```python
from build123d import *

# Parameters (mm, degrees)
SKETCH1_W         = 18
SKETCH1_H         = 42.5
IDCHAMFER_SIZE    = 2
ODCHAMFER_SIZE    = 4.5
IDCHAMFERFAR_SIZE = 2


with BuildPart() as part:
    # Sketch1 → Base-Revolve (revolve)
    with BuildSketch(Plane.XY, mode=Mode.PRIVATE) as base_revolve_sk:
        with Locations((-9, 103.75)):
            Rectangle(SKETCH1_W, SKETCH1_H)
    revolve(base_revolve_sk.sketch.rotate(Axis((-34.925, 0, 0), (1, 0, 0)), 90), axis=Axis((-34.925, 0, 0), (1, 0, 0)))

    # IDChamfer
    idchamfer_edges = [part.edges().sort_by_distance(p)[0] for p in [
        (0, 0, -82.5),
    ]]
    chamfer(idchamfer_edges, length=IDCHAMFER_SIZE)

    # ODChamfer
    odchamfer_edges = [part.edges().sort_by_distance(p)[0] for p in [
        (0, 0, -125),
    ]]
    chamfer(odchamfer_edges, length=ODCHAMFER_SIZE)

    # IDChamferFar
    idchamferfar_edges = [part.edges().sort_by_distance(p)[0] for p in [
        (-18, 0, -82.5),
    ]]
    chamfer(idchamferfar_edges, length=IDCHAMFERFAR_SIZE)


solid = part.part
```
Can you work these out from the model? Positions are in its coordinate system, mm. Give positions to 0.01 mm unless a question says otherwise; leave off trailing zeros. Loops run counter-clockwise (first coordinate to the right, second up) from the corner with the lowest first, then second, coordinate; pieces in that order, holes last. Notation, with made-up numbers: M 35,-5.75 L 69,-5.75 A33 ccw 69,22.25 Z; hole C 88,55.5 d7. An arc over 180 degrees is marked long. Answer in a Markdown table with one row per item.
1. Thinking about a two-plate mould opening in Z: for faces 1 (the cylindrical face through (-8.9, 80.54, -17.88)), 2 (the conical face through (-0.28, -36.28, 115.2)), 3 (the conical face through (-1.875, -24.818, 78.81)), 4 (the flat face through (0, 25, 82)), which applies, released by +Z, released by -Z, zero draft, split by the parting line, or undercut?
Taken from the geometry:
| item | result |
|---|---|
| face 1 | undercut |
| face 2 | split by the parting line |
| face 3 | undercut |
| face 4 | zero draft |
2. If I drill on line 1 along Y through (x, z) = (-6.25, 0); line 2 along Y through (x, z) = (-2.25, 20); line 3 along Z through (x, y) = (-7, -39), over which ranges is the centre line in solid material (lowest first)?
Taken from the geometry:
| item | result |
|---|---|
| line 1 | y = -125 to -82.5, 82.5 to 125 |
| line 2 | y = -121.11 to -80.04, 80.04 to 121.11 |
| line 3 | z = -118.76 to -72.7, 72.7 to 118.76 |
3. Suppose I cut it at A-A on y = 0. Write out the boundary of the cut face in (x, z), plus the area to 3 significant figures.
Taken from the geometry:
| item | result |
|---|---|
| outline | M -18,-125 L -4.5,-125 L 0,-120.5 L 0,-84.5 L -2,-82.5 L -16,-82.5 L -18,-84.5 Z; M -18,84.5 L -16,82.5 L -2,82.5 L 0,84.5 L 0,120.5 L -4.5,125 L -18,125 Z |
| area | 1,500 mm² |
4. For pin 1 Ø1 at (x, z) = (-13, -99) entering from -Y; pin 2 Ø1 at (x, y) = (-11.5, 37.5) entering from +Z; pin 3 Ø3 at (x, y) = (-11.5, 41) entering from +Z, each with a flat end and sliding along its axis, tell me the tip position at first contact or that it passes through.
Taken from the geometry:
| item | result |
|---|---|
| pin 1 | stops at y = -76.96 |
| pin 2 | stops at z = 119.4 |
| pin 3 | stops at z = 118.59 |
5. Suppose I cut it at C-C on x = -12.5. Write out the boundary of the cut face in (y, z), plus the area to 3 significant figures.
Taken from the geometry:
| item | result |
|---|---|
| outline | C 0,0 d250; hole C 0,0 d165 |
| area | 27,700 mm² |
